Could you check a few things on this model? Use its own coordinates, in mm. A direction names the side the tool comes from. Give positions to 0.01 mm unless a question says otherwise; leave off trailing zeros. Write each loop counter-clockwise with the first axis right and the second up, starting at its lowest first coordinate (ties: lowest second). Pieces come first, ordered by that corner, then holes. Notation, with made-up numbers: (87.25, 46) -> (132.25, 46) arc R17 ccw to (132.25, 69) -> close; hole circle Ø3 at (-12, 34). An arc over 180 degrees is marked (long way). Write item = value, one per line. Start each with the question number.
```python
from build123d import *

# Parameters (mm, degrees)
ESBO_O1_W                = 8
ESBO_O1_H                = 2
RESSALTO_EXTRUS_O1_DEPTH = 10
CORTE_EXTRUS_O1_REACH    = 75.763
ESBO_O4_W                = 20
ESBO_O4_H                = 15
ESBO_O4_R                = 2
RESSALTO_EXTRUS_O2_DEPTH = 5
ESBO_O5_R                = 1.65
RESSALTO_EXTRUS_O3_DEPTH = 5


with BuildPart() as part:
    # Esboço1 → Ressalto-extrusão1 (new, symmetric)
    with BuildSketch(Plane(origin=(0, 0, 0), x_dir=(0, 0, -1), z_dir=(1, 0, 0))):
        Polygon((-35, 21), (-10, 21), (-10, 5), (10, 5), (10, 21), (35, 21), (35, 0), (-35, 0), align=None)
        with Locations((-22.5, 4)):
            Rectangle(ESBO_O1_W, ESBO_O1_H, mode=Mode.SUBTRACT)
        with Locations((22.5, 4)):
            Rectangle(ESBO_O1_W, ESBO_O1_H, mode=Mode.SUBTRACT)
    extrude(amount=RESSALTO_EXTRUS_O1_DEPTH, both=True)

    # Corte-extrusão1: up to this face of the body (flat: up to its plane)
    corte_extrus_o1_end = Plane(part.part.faces().sort_by_distance((0, 10.5, -35))[0])
    # Esboço2 → Corte-extrusão1 (cut, up to the picked face)
    with BuildSketch(Plane.XY.offset(35), mode=Mode.PRIVATE) as corte_extrus_o1_sk1:
        with BuildLine():
            Line((-6.873863542, 21), (6.873863542, 21))
            ThreePointArc((6.873863542, 21), (0, 10.5), (-6.873863542, 21))
        make_face()
    corte_extrus_o1_tool1 = split(extrude(corte_extrus_o1_sk1.sketch, amount=-CORTE_EXTRUS_O1_REACH, mode=Mode.PRIVATE), bisect_by=corte_extrus_o1_end, keep=Keep.BOTH, mode=Mode.PRIVATE)
    add(corte_extrus_o1_tool1.solids().sort_by(Axis((0, 16.361219, 35), (0, 0, -1)))[0], mode=Mode.SUBTRACT)

    # Esboço4 → Ressalto-extrusão2 (add)
    # profile 1 of 2: a face of its own
    with BuildSketch(Plane(origin=(0, 5, 0), x_dir=(1, 0, 0), z_dir=(0, 1, 0))):
        with Locations((0, 42.5)):
            Rectangle(ESBO_O4_W, ESBO_O4_H)
        with Locations(Location((0, 42.5, 0), (0, 0, 270))):
            Circle(ESBO_O4_R, mode=Mode.SUBTRACT)
    # profile 2 of 2: a face of its own
    with BuildSketch(Plane(origin=(0, 5, 0), x_dir=(1, 0, 0), z_dir=(0, 1, 0))):
        with Locations((0, -42.5)):
            Rectangle(ESBO_O4_W, ESBO_O4_H)
        with Locations(Location((0, -42.5, 0), (0, 0, 270))):
            Circle(ESBO_O4_R, mode=Mode.SUBTRACT)
    extrude(amount=-RESSALTO_EXTRUS_O2_DEPTH)

    # Esboço5 → Ressalto-extrusão3 (add)
    with BuildSketch(Plane.XZ):
        with BuildLine():
            Line((18, 17.5), (10, 17.5))
            Line((10, 17.5), (10, -17.5))
            Line((10, -17.5), (18, -17.5))
            ThreePointArc((18, -17.5), (21.889087297, -15.889087297), (23.5, -12))
            Line((23.5, -12), (23.5, 12))
            ThreePointArc((23.5, 12), (21.889087297, 15.889087297), (18, 17.5))
        make_face()
        with Locations(Location((18, 12, 0), (0, 0, 270))):
            Circle(ESBO_O5_R, mode=Mode.SUBTRACT)
        with Locations(Location((18, -12, 0), (0, 0, 270))):
            Circle(ESBO_O5_R, mode=Mode.SUBTRACT)
    extrude(amount=-RESSALTO_EXTRUS_O3_DEPTH)


solid = part.part
```
(1) If I drill on line 1 along X through (y, z) = (18.5, -17.5); line 2 along Z through (x, y) = (-8, 16); line 3 along X through (y, z) = (3.05, -42.5), over which ranges is the centre line in solid material (lowest first)? Write a range as from..to.
(2) We'd pull the mould along Z, two halves only. Please class faces 5 (the flat face through (10, 11, -25)), 6 (the cylindrical face through (19.39, 2.46, 11.11)), 7 (the cylindrical face through (21.85, 2.46, -15.93)): released by +Z, released by -Z, zero draft, split by the parting line, or undercut.
(3) Imagine slicing it at C-C (y = 7.5). Please give me the cut outline in (x, z).
(4) Imagine slicing it at D-D (z = -7). Please give me the cut outline in (x, y).
(5) On a 3-axis mill with a long thin cutter (end or side, diameter ignored), from which of +Z, -Z, +X, -X, +Y, -Y can I reach the whole of each face in a straight line? I mean faces 1 (the flat face through (0, 9, 35)), 2 (the flat face through (0, 4, -18.5)), 3 (the flat face through (0, 9, -10)), 4 (the flat face through (-8, 21, 23)). Say none if no direction works.
(6) Imagine slicing it at A-A (y = 15). Please give me the cut outline in (x, z), then the cut area to 3 significant figures.
(7) I'm going to push flat-ended pins straight in: pin 1 (2 mm diameter, centred on x = 18, z = 12, fed in from -Y); pin 2 (8 mm diameter, centred on x = -3.5, y = 15, fed in from +Z); pin 3 (1.5 mm diameter, centred on x = 12.5, y = 2, fed in from +Z); pin 4 (6.5 mm diameter, centred on y = 6, z = 39.5, fed in from +X). Where does each tip first touch, or does it pass through?
(8) Imagine slicing it at B-B (z = 42.5). Please give me the cut outline in (x, y).
Answers below:
q1.line_1 = -10..-7.48, 7.48..10
q1.line_2 = -35..-10, 10..35
q1.line_3 = -10..-2, 2..10
q2.face_5 = zero draft
q2.face_6 = undercut
q2.face_7 = released by -Z
q3.outline = (-10, -35) -> (10, -35) -> (10, -10) -> (-10, -10) -> close; (-10, 10) -> (10, 10) -> (10, 35) -> (-10, 35) -> close
q4.outline = (-10, 0) -> (23.5, 0) -> (23.5, 5) -> (-10, 5) -> close
q5.face_1 = +Z, +X, -X, +Y
q5.face_2 = +X, -X
q5.face_3 = +X, -X, +Y
q5.face_4 = +Z, -Z, +X, -X, +Y
q6.outline = (-10, -35) -> (-6.87, -35) -> (-6.87, -10) -> (-10, -10) -> close; (-10, 10) -> (-6.87, 10) -> (-6.87, 35) -> (-10, 35) -> close; (6.87, -35) -> (10, -35) -> (10, -10) -> (6.87, -10) -> close; (6.87, 10) -> (10, 10) -> (10, 35) -> (6.87, 35) -> close
q6.area = 313 mm^2
q7.pin_1 = through
q7.pin_2 = 35
q7.pin_3 = 17.5
q7.pin_4 = 10
q8.outline = (-10, 0) -> (-2, 0) -> (-2, 5) -> (-10, 5) -> close; (2, 0) -> (10, 0) -> (10, 5) -> (2, 5) -> close
